Part model, mm, in its own coordinate system. Face numbers are marked on the shaded views. A direction names the side the tool comes from. Round coordinates to 2 decimals unless told otherwise and drop trailing zeros. Write each loop counter-clockwise with the first axis right and the second up, starting at its lowest first coordinate (ties: lowest second). Pieces come first, ordered by that corner, then holes. Notation, with made-up numbers: M 82,-28 L 110,-28 A20 ccw 110,-12 Z; hole C 42,66 d5. An arc over 180 degrees is marked long. Use a Markdown table: item, result. Add a question column.
1) Drop flat-ended pins along their axis: P1, Ø1, axis at y = -1.5, z = -6.5, coming from the -X side; P2, Ø1.5, axis at x = 0, z = -5.5, coming from the +Y side (3 decimals); P3, Ø6, axis at x = -4.5, y = -5, coming from the -Z side. Give the stop position or say it passes through.
2) Which spindle directions (+Z, -Z, +X, -X, +Y, -Y) get a long thin tool onto all of the face, cutting with end or side? Do the marked faces 1 and 2. Say none if no direction does.
3) Slice it at C-C on z = -3.5. Write the cut outline in (x, y) (3 decimals), plus the area to 3 significant figures.
4) Wall check: probe 1 along Z at (x, y) = (-0.5, 3.25); probe 2 along Y at (x, z) = (-1, -1.5); probe 3 along X at (y, z) = (1.5, -4.25). Give the ranges that are in metal, low to high.
5) Slice it at A-A on y = 0. Write the cut outline in (x, z) (3 decimals).
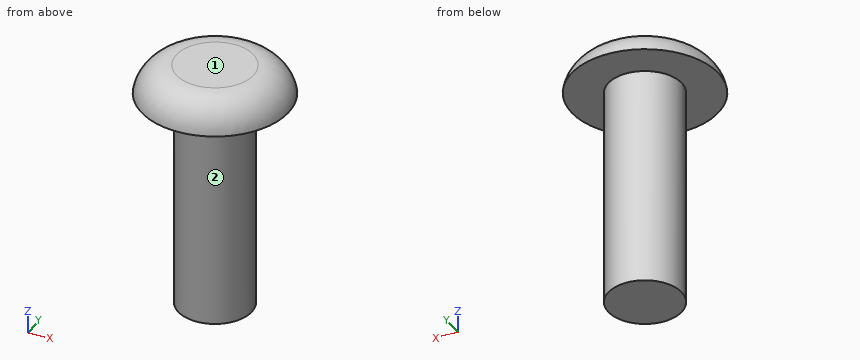
```python
from build123d import *

# Parameters (mm, degrees)
F0_R     = 6.35
F1_DEPTH = 2.54
F3_R     = 3.175
F4_DEPTH = 19.05


# Not quite as in the source:
# - a fillet or chamfer that OpenCascade refuses, or shapes differently, is made with other operations: its cross-section is extruded or revolved along the edge and cut away or added


with BuildPart() as f1:
    # F0 (on Top) → F1 (new body)
    with BuildSketch(Plane.XY):
        Circle(F0_R)
    extrude(amount=F1_DEPTH)

    # F2: fillet of radius 3.0660512242 on 1 edges, made by hand

    # F2_s1 → F2_t2 (revolve, cut)
    with BuildSketch(Plane.XZ):
        with BuildLine():
            ThreePointArc((6.35, 0), (5.3027068749, 1.8206027884), (3.3294139279, 2.54))
            Line((3.3294139279, 2.54), (6.35, 2.54))
            Line((6.35, 2.54), (6.35, 0))
        make_face()
    revolve(axis=Axis((0, 0, 2.54), (0, 0, 1)), mode=Mode.SUBTRACT)

    # F3 (on face) → F4 (join)
    with BuildSketch(Plane(origin=(0, 0, 0), x_dir=(1, 0, 0), z_dir=(0, 0, -1))):
        Circle(F3_R)
    extrude(amount=F4_DEPTH)


solid = f1.part
```
Entries:
| question | item | result |
|---|---|---|
| 1 | P1 | stops at x = -3.01 |
| 1 | P2 | stops at y = 3.175 |
| 1 | P3 | stops at z = 0 |
| 2 | face 1 | +Z, +X, -X, +Y, -Y |
| 2 | face 2 | -Z |
| 3 | outline | C 0,0 d6.35 |
| 3 | area | 31.7 mm^2 |
| 4 | probe 1 | z = 0 to 2.54 |
| 4 | probe 2 | y = -3.01 to 3.01 |
| 4 | probe 3 | x = -2.8 to 2.8 |
| 5 | outline | M -6.35,0 L -3.175,0 L -3.175,-19.05 L 3.175,-19.05 L 3.175,0 L 6.35,0 A3.066 ccw 3.329,2.54 L -3.329,2.54 A3.066 ccw Z |
